Part model, mm, in its own coordinate system. Face numbers are marked on the shaded views. A direction names the side the tool comes from. Give positions to 0.01 mm unless a question says otherwise; leave off trailing zeros. Order: outer loops, then holes, each group sorted by start corner. A loop starts at its lowest first (then second) coordinate and runs counter-clockwise, first axis right, second up. Notation, with made-up numbers: (-1.5, 68.5) - (44.5, 68.5) arc R13 cw to (44.5, 89.5) - close; hole circle Ø5 at (28, 6). An arc over 180 degrees is marked (long way). One line per item, written item: value.
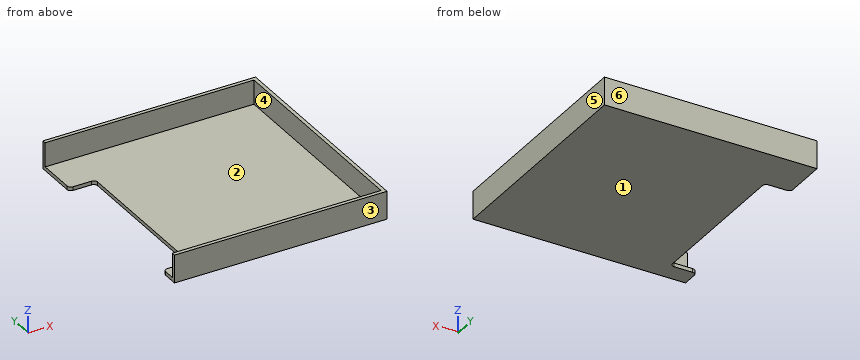
```python
from build123d import *

# Parameters (mm, degrees)
BOX070_W     = 1.4
BOX070_H     = 8.6
BOX070_DEPTH = 0.2
FILLET018_R  = 0.2
BOX069_W     = 11.2
BOX069_H     = 11.6
BOX069_DEPTH = 1.3
BOX068_W     = 11.4
BOX068_H     = 12
BOX068_DEPTH = 1.5
FILLET019_R  = 0.2


with BuildPart() as fillet020:
    # Box070 → Box070 (new body)
    with BuildSketch(Plane(origin=(0, 1, 0), x_dir=(1, 0, 0), z_dir=(0, 0, 1))):
        with Locations((0.7, 4.3)):
            Rectangle(BOX070_W, BOX070_H)
    extrude(amount=BOX070_DEPTH)

    # Fillet018
    fillet018_edges = [fillet020.edges().sort_by_distance(p)[0] for p in [
        (1.4, 1, 0.1),
        (1.4, 9.6, 0.1),
    ]]
    fillet(fillet018_edges, radius=FILLET018_R)


with BuildPart() as fusion052:
    # Box069 → Box069 (new body)
    with BuildSketch(Plane(origin=(0, 0.2, 0.2), x_dir=(1, 0, 0), z_dir=(0, 0, 1))):
        with Locations((5.6, 5.8)):
            Rectangle(BOX069_W, BOX069_H)
    extrude(amount=BOX069_DEPTH)

    # Fusion052: union Fillet020
    add(fillet020.part)


with BuildPart() as sd_card_slot:
    # Box068 → Box068 (new body)
    with BuildSketch(Plane.XY):
        with Locations((5.7, 6)):
            Rectangle(BOX068_W, BOX068_H)
    extrude(amount=BOX068_DEPTH)

    # Cut017: cut Fusion052
    add(fusion052.part, mode=Mode.SUBTRACT)

    # Fillet019
    fillet019_edges = [sd_card_slot.edges().sort_by_distance(p)[0] for p in [
        (0, 1, 0.1),
        (0, 9.6, 0.1),
    ]]
    fillet(fillet019_edges, radius=FILLET019_R)


with BuildPart() as sd_card_slot_1:
    # Fillet019 placement: moved
    add(sd_card_slot.part.moved(Location((1.7, 22, -1.5))))


solid = sd_card_slot_1.part
```
1) Slice it at D-D on y = 29.75. Write the cut outline in (x, z).
Answer:
outline: (3.1, -1.5) - (13.1, -1.5) - (13.1, 0) - (12.9, 0) - (12.9, -1.3) - (3.1, -1.3) - close
2) Drop a flat-ended pin along its axis: P1, Ø1.5, axis at x = 10, y = 24.5, coming from the +Z side. Give the stop position or say it passes through.
Answer:
P1: stops at z = -1.3
3) Which spindle directions (+Z, -Z, +X, -X, +Y, -Y) get a long thin tool onto all of the face, cutting with end or side? Do the marked faces 1 and 2. Say none if no direction does.
Answer:
face 1: -Z, +X, -X, +Y, -Y
face 2: +Z, -X
4) Two-plate mould, pull along Y, no slides. Class the marked faces 3, 4, 5 and 6: pulls with the +Y half, pulls with the -Y half, needs draft (parallel to the pull), parting line crosses it, or undercut.
Answer:
face 3: pulls with the -Y half
face 4: undercut
face 5: needs draft
face 6: pulls with the +Y half
5) Slice it at A-A on x = 5. Write the cut outline in (y, z), then the cut area to 3 significant figures.
Answer:
outline: (22, -1.5) - (34, -1.5) - (34, 0) - (33.8, 0) - (33.8, -1.3) - (22.2, -1.3) - (22.2, 0) - (22, 0) - close
area: 2.92 mm2
6) Slice it at B-B on y = 32.5. Write the cut outline in (x, z), then the cut area to 3 significant figures.
Answer:
outline: (1.7, -1.5) - (13.1, -1.5) - (13.1, 0) - (12.9, 0) - (12.9, -1.3) - (1.7, -1.3) - close
area: 2.54 mm2
7) Slice it at C-C on z = -0.45. Write the cut outline in (x, y), then the cut area to 3 significant figures.
Answer:
outline: (1.7, 22) - (13.1, 22) - (13.1, 34) - (1.7, 34) - (1.7, 33.8) - (12.9, 33.8) - (12.9, 22.2) - (1.7, 22.2) - close
area: 6.88 mm2
8) Wall check: line 1 along Y through (x, z) = (12.25, -0.55); line 2 along X through (y, z) = (28.5, -0.75); line 3 along Z through (x, y) = (9.25, 28.75). Give the ranges that are in metal, low to high. Write a range as [from, to].
Answer:
line 1: y = [22, 22.2], [33.8, 34]
line 2: x = [12.9, 13.1]
line 3: z = [-1.5, -1.3]
